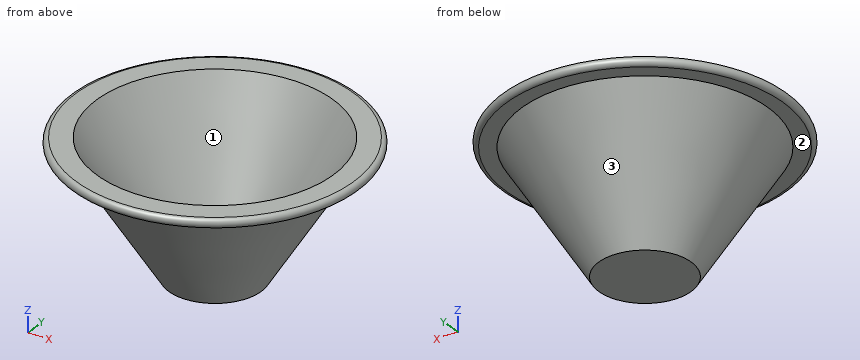
Autodesk Fusion 360 part; units mm, degrees
sketch "Sketch1" plane through (0, 0, 0) normal (0, 1, 0) x (1, 0, 0) in component "bowl"
  line L0 (0, 0) -> (15, 0)
  line L1 (15, 0) -> (40, -40)
  line L2 (40, -40) -> (45, -40)
  line L3 (0, -3) -> (13.3373, -3)
  line L4 (13.3373, -3) -> (38.3373, -43)
  line L5 (38.3373, -43) -> (45, -43)
  arc A0 (45, -43) -> (45, -40) centre (45, -41.5) ccw
  line L6 (0, -3) -> (0, 0)
  dimension "d1" = 3
revolve "Revolve1" add sketch "Sketch1" angle 360 about axis through (0, 0, 1.75) along (0, 0, 1) in component "bowl"
component "bowl" placed x (1, 0, 0) y (0, 1, 0) z (0, 0, 1) at (0, 0, 0)
Design review of the part built by this model. Coordinates are the model's own, in mm. Face numbers are marked on the shaded views. Coordinates: 2 decimals unless noted, no trailing zeros. Write each loop counter-clockwise with the first axis right and the second up, starting at its lowest first coordinate (ties: lowest second). Pieces come first, ordered by that corner, then holes. Notation, with made-up numbers: (81.25, 84) -> (123.25, 84) arc R32 ccw to (123.25, 122) -> close; hole circle Ø2 at (54.5, 25). An arc over 180 degrees is marked (long way). Write each question's results on one line, items separated by ' | '. Start each with the question number.
(1) Take a section at A-A on y = 0. Write out the cut boundary in (x, z).
(2) For line 1 along Y through (x, z) = (-20.5, 39); line 2 along Y through (x, z) = (4.5, 34); line 3 along X through (y, z) = (-20.5, 18), list the stretches that pass through material, from the lowest coordinate up. Write a range as from..to.
(3) Take a section at C-C on z = 8. Write out the cut boundary in (x, y), and give its area (3 significant figures).
(4) Clearance check with flat-ended pins moving along their axes: P1, Ø1, axis at x = 32, y = 32.5, coming from the -Z side; P2, Ø21.5, axis at x = -1, y = 2, coming from the +Z side; P3, Ø4, axis at x = -36, y = 33, coming from the +Z side; P4, Ø1, axis at x = -20.5, y = -1.5, coming from the +Z side. State where each tip first meets the part, or that it passes through.
(5) The part is to be moulded in two halves that separate along Y. For the marked faces 1, 2 and 3, say which applies: pulls with the +Y half, pulls with the -Y half, needs draft (parallel to the pull), parting line crosses it, or undercut.
Results found:
1) outline: (-45, 40) -> (-40, 40) -> (-15, 0) -> (15, 0) -> (40, 40) -> (45, 40) arc R1.5 ccw to (45, 43) -> (38.34, 43) -> (13.34, 3) -> (-13.34, 3) -> (-38.34, 43) -> (-45, 43) arc R1.5 ccw to start
2) line 1: y = -33.62..-29.39, 29.39..33.62 | line 2: y = -35.97..-32.4, 32.4..35.97 | line 3: x = -16.4..-9.78, 9.78..16.4
3) outline: circle Ø40 at (0, 0); hole circle Ø32.92 at (0, 0) | area: 405 mm2
4) P1: stops at z = 40 | P2: stops at z = 3 | P3: passes through | P4: stops at z = 15.35
5) face 1: undercut | face 2: needs draft | face 3: parting line crosses it
